```python
from build123d import *

# Parameters (mm, degrees)
SKETCH1_W           = 25
SKETCH1_H           = 20
BOSS_EXTRUDE1_DEPTH = 1.5
SKETCH2_W           = 28
SKETCH2_H           = 23
SKETCH2_W_2         = 25
SKETCH2_H_2         = 20
BOSS_EXTRUDE2_DEPTH = 11.5
SKETCH3_W           = 15.8
SKETCH3_H           = 4
CUT_EXTRUDE1_DEPTH  = 10


with BuildPart() as part:
    # Sketch1 → Boss-Extrude1 (new body)
    with BuildSketch(Plane(origin=(0, 0, 0), x_dir=(1, 0, 0), z_dir=(0, 1, 0))):
        with Locations((12.5, 10)):
            Rectangle(SKETCH1_W, SKETCH1_H)
    extrude(amount=BOSS_EXTRUDE1_DEPTH)

    # Sketch2 → Boss-Extrude2 (add)
    with BuildSketch(Plane.XZ):
        with Locations((12.5, -10)):
            Rectangle(SKETCH2_W, SKETCH2_H)
        with Locations((12.5, -10)):
            Rectangle(SKETCH2_W_2, SKETCH2_H_2, mode=Mode.SUBTRACT)
    extrude(amount=-BOSS_EXTRUDE2_DEPTH)

    # Sketch3 → Cut-Extrude1 (cut)
    with BuildSketch(Plane.ZY.offset(-25)):
        with Locations((-9.1, 6)):
            Rectangle(SKETCH3_W, SKETCH3_H)
    extrude(amount=-CUT_EXTRUDE1_DEPTH, mode=Mode.SUBTRACT)


solid = part.part
```
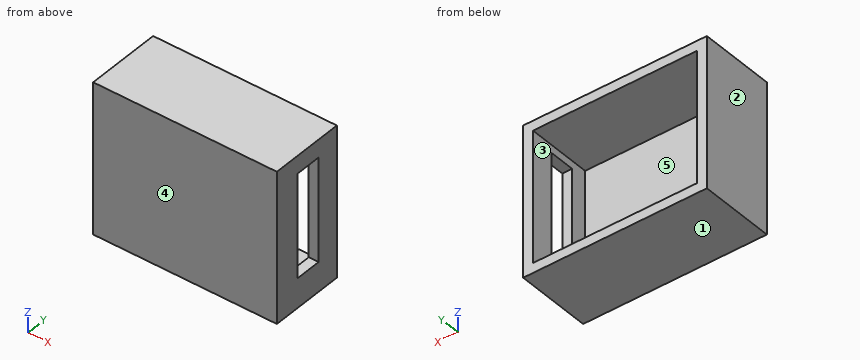
Design review of the part built by this model. Coordinates are the model's own, in mm. Face numbers are marked on the shaded views. A direction names the side the tool comes from. Give positions to 0.01 mm unless a question says otherwise; leave off trailing zeros. Order: outer loops, then holes, each group sorted by start corner. A loop starts at its lowest first (then second) coordinate and runs counter-clockwise, first axis right, second up. Notation, with made-up numbers: (43.5, 58) -> (73.5, 58) arc R31 ccw to (73.5, 85) -> close; hole circle Ø8 at (-14, 47). An arc over 180 degrees is marked (long way). Write item = value, one per line. Start each with the question number.
(1) To check wall thickness, follow line 1 along Z through (x, y) = (20, 8.75); line 2 along X through (y, z) = (10.5, -5.5); line 3 along Y through (x, z) = (10.5, -13.5). State the ranges of each line that lie inside material, in increasing order.
(2) We need section B-B on y = 10.25. Write out the cut boundary in (x, z), plus the area to 3 significant figures.
(3) We need section D-D on z = -19.5. Write out the cut boundary in (x, y).
(4) We need section A-A on z = -11.5. Write out the cut boundary in (x, y).
(5) We need section C-C on x = 3.5. Write out the cut boundary in (y, z), plus the area to 3 significant figures.
(6) Mouldability with a two-part tool opening along Z and no side actions: class the marked faces 1, 2 and 3 as +Z half, -Z half, draft (parallel to the pull), parting line (faces both ways), or undercut.
(7) For the marked faces 4 and 5, list the 3-axis set-ups (+Z, -Z, +X, -X, +Y, -Y) from which the entire face can be reached by the end or side of a thin tool; tool diameter is ignored.
Numbers:
q1.line_1 = -21.5 to -20, 0 to 1.5
q1.line_2 = -1.5 to 0, 25 to 26.5
q1.line_3 = 0 to 1.5
q2.outline = (-1.5, -21.5) -> (26.5, -21.5) -> (26.5, 1.5) -> (-1.5, 1.5) -> close; hole (0, -20) -> (25, -20) -> (25, 0) -> (0, 0) -> close
q2.area = 144 mm^2
q3.outline = (-1.5, 0) -> (26.5, 0) -> (26.5, 11.5) -> (25, 11.5) -> (25, 1.5) -> (0, 1.5) -> (0, 11.5) -> (-1.5, 11.5) -> close
q4.outline = (-1.5, 0) -> (26.5, 0) -> (26.5, 4) -> (25, 4) -> (25, 1.5) -> (0, 1.5) -> (0, 11.5) -> (-1.5, 11.5) -> close; (25, 8) -> (26.5, 8) -> (26.5, 11.5) -> (25, 11.5) -> close
q5.outline = (0, -21.5) -> (11.5, -21.5) -> (11.5, -20) -> (1.5, -20) -> (1.5, 0) -> (11.5, 0) -> (11.5, 1.5) -> (0, 1.5) -> close
q5.area = 64.5 mm^2
q6.face_1 = -Z half
q6.face_2 = draft
q6.face_3 = undercut
q7.face_4 = +Z, -Z, +X, -X, -Y
q7.face_5 = +Y
